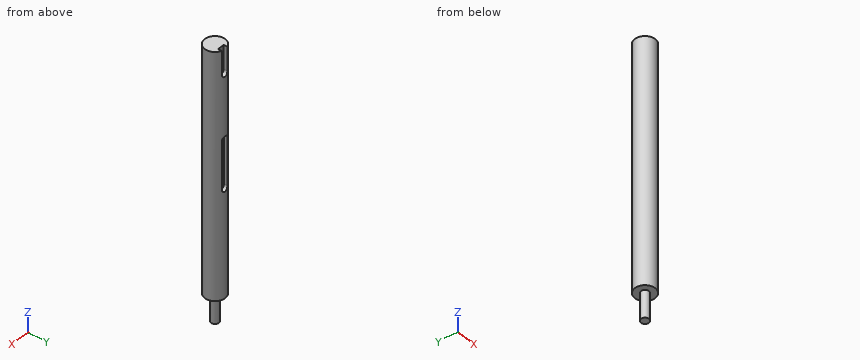
from build123d import *

# Parameters (mm, degrees)
SKETCH1_R           = 7.5
BOSS_EXTRUDE1_DEPTH = 200
SKETCH2_R           = 7.5
SKETCH2_R_2         = 3
CUT_EXTRUDE1_DEPTH  = 20
CUT_EXTRUDE3_START  = 10
CUT_EXTRUDE3_DEPTH  = 12.5
CUT_EXTRUDE4_START  = 10
CUT_EXTRUDE4_DEPTH  = 12.7


with BuildPart() as part:
    # Sketch1 → Boss-Extrude1 (new body)
    with BuildSketch(Plane.XY):
        Circle(SKETCH1_R)
    extrude(amount=BOSS_EXTRUDE1_DEPTH)

    # Sketch2 → Cut-Extrude1 (cut)
    with BuildSketch(Plane(origin=(0, 0, 0), x_dir=(-1, 0, 0), z_dir=(0, 0, -1))):
        Circle(SKETCH2_R)
        Circle(SKETCH2_R_2, mode=Mode.SUBTRACT)
    extrude(amount=-CUT_EXTRUDE1_DEPTH, mode=Mode.SUBTRACT)

    # Sketch5 → Cut-Extrude3 (cut)
    with BuildSketch(Plane(origin=(0, 7.071067812, 0), x_dir=(1, 0, 0), z_dir=(0, 1, 0)).offset(CUT_EXTRUDE3_START)):
        with BuildLine():
            Line((2.5, -99.5781), (2.5, -134.5781))
            ThreePointArc((2.5, -134.5781), (0, -137.0781), (-2.5, -134.5781))
            Line((-2.5, -134.5781), (-2.5, -99.5781))
            ThreePointArc((-2.5, -99.5781), (0, -97.0781), (2.5, -99.5781))
        make_face()
    extrude(amount=-CUT_EXTRUDE3_DEPTH, mode=Mode.SUBTRACT)

    # Sketch6 → Cut-Extrude4 (cut)
    with BuildSketch(Plane(origin=(0, 7.071067812, 0), x_dir=(1, 0, 0), z_dir=(0, 1, 0)).offset(CUT_EXTRUDE4_START)):
        with BuildLine():
            Line((-2.5, -200), (-2.5, -182.5))
            ThreePointArc((-2.5, -182.5), (0, -180), (2.5, -182.5))
            Line((2.5, -182.5), (2.5, -200))
            ThreePointArc((2.5, -200), (0, -202.5), (-2.5, -200))
        make_face()
    extrude(amount=-CUT_EXTRUDE4_DEPTH, mode=Mode.SUBTRACT)


solid = part.part
Read the model definition and answer for the solid it produces. Units are mm, in the model's axes. Coordinates: 2 decimals unless noted, no trailing zeros. Loops run counter-clockwise (first coordinate to the right, second up) from the corner with the lowest first, then second, coordinate; pieces in that order, holes last. Notation, with made-up numbers: (-13, 57) -> (5, 57) arc R16 cw to (5, 73) -> close; hole circle Ø3 at (66.5, -21). An arc over 180 degrees is marked (long way). Write item = value, one per line. Start each with the question number.
1) The part is cut by section C-C, the plane z = 144. Determine the outline of the cut face in (x, y), plus the area to 3 significant figures.
2) Find the intervals of material crossed by L1, parallel to Y at x = 0.75, z = 81; L2, parallel to Z at x = -4.75, y = -4.25; L3, parallel to X at y = 5.25, z = 186, in increasing order. Write a range as from..to.
3) The part is cut by section B-B, the plane x = 0. Determine the outline of the cut face in (y, z), plus the area to 3 significant figures.
4) The part is cut by section D-D, the plane z = 123. Determine the outline of the cut face in (x, y).
5) Given P1, Ø4, axis at y = -6, z = 137, coming from the +X side; P2, Ø5, axis at x = -4, y = -5, coming from the -Z side; P3, Ø2, axis at y = 6, z = 194.5, coming from the +X side, each flat-ended and moving along its own axis, determine where each tip first touches the part or whether it passes through.
6) The part is cut by section A-A, the plane y = 0. Determine the outline of the cut face in (x, z), plus the area to 3 significant figures.
Result:
q1.outline = circle Ø15 at (0, 0)
q1.area = 177 mm²
q2.L1 = -7.46..7.46
q2.L2 = 20..200
q2.L3 = -5.36..-2.5, 2.5..5.36
q3.outline = (-7.5, 20) -> (-3, 20) -> (-3, 0) -> (3, 0) -> (3, 20) -> (7.5, 20) -> (7.5, 97.08) -> (4.57, 97.08) -> (4.57, 137.08) -> (7.5, 137.08) -> (7.5, 180) -> (4.37, 180) -> (4.37, 200) -> (-7.5, 200) -> close
q3.area = 2,640 mm²
q4.outline = (-2.5, 4.57) -> (-2.5, 7.07) arc R7.5 ccw (long way) to (2.5, 7.07) -> (2.5, 4.57) -> close
q5.P1 = 6.34
q5.P2 = 20
q5.P3 = 5.59
q6.outline = (-7.5, 20) -> (-3, 20) -> (-3, 0) -> (3, 0) -> (3, 20) -> (7.5, 20) -> (7.5, 200) -> (-7.5, 200) -> close
q6.area = 2,820 mm²
